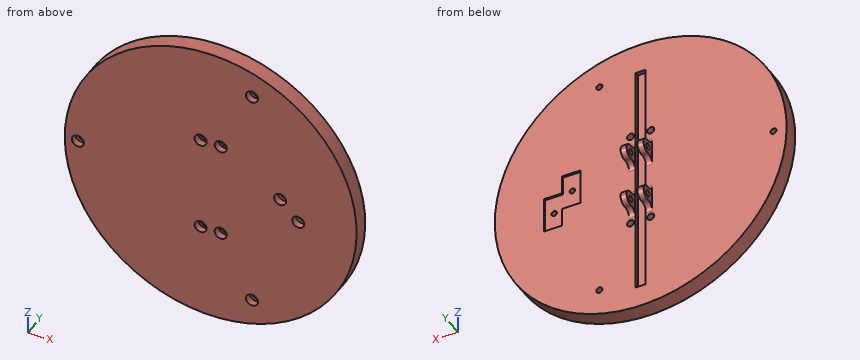
```python
from build123d import *

# Parameters (mm, degrees)
SKETCH_1_R             = 72.5
EXTRUDE_1_DEPTH        = 8
SKETCH_4_R             = 1.75
CUT_EXTRUDE_4_DEPTH    = 10
CUT_EXTRUDE_2_REACH    = 104.842
SKETCH_6_R             = 1.5
SKETCH_10_R            = 1.5
CUT_EXTRUDE_6_DEPTH    = 10
SKETCH_8_W             = 3
SKETCH_8_H             = 7
EXTRUDE_2_DEPTH        = 8
FILLET_1_R             = 3.5
SKETCH_9_R             = 1.5
CUT_EXTRUDE_5_DEPTH    = 106.675399219
FILLET_1_OF_MIRROR_1_R = 3.5
MIRROR_START           = -5.7
MIRROR_2_OUTLINE_R     = 1.5
MIRROR_2_DEPTH         = 3
SKETCH_11_R            = 1.35
CUT_EXTRUDE_7_DEPTH    = 103.842111997
SKETCH_12_W            = 9
SKETCH_12_H            = 18
CUT_EXTRUDE_8_DEPTH    = 1
SKETCH_7_R             = 3
CUT_EXTRUDE_3_DEPTH    = 3.5
SKETCH_14_W            = 5
SKETCH_14_H            = 1
SKETCH_14_H_2          = 117.17646446
CUT_EXTRUDE_9_DEPTH    = 2


# Read off the part's stored shape, not the designer's step: 镜向2
with BuildPart() as part:
    # 草图1 → 凸台-拉伸1 (new body)
    with BuildSketch(Plane(origin=(0, 0, 0), x_dir=(1, 0, 0), z_dir=(0, 1, 0))):
        with Locations(Location((0, 0, 0), (0, 0, 270))):
            Circle(SKETCH_1_R)
    extrude(amount=EXTRUDE_1_DEPTH)

    # 草图4 → 切除-拉伸4 (cut)
    with BuildSketch(Plane(origin=(0, 8, 0), x_dir=(1, 0, 0), z_dir=(0, 1, 0))):
        with Locations(Location((-5, -23, 0), (0, 0, 270))):
            Circle(SKETCH_4_R)
        with Locations(Location((-5, 25, 0), (0, 0, 270))):
            Circle(SKETCH_4_R)
        with Locations(Location((5, 25, 0), (0, 0, 270))):
            Circle(SKETCH_4_R)
        with Locations(Location((5, -23, 0), (0, 0, 270))):
            Circle(SKETCH_4_R)
    extrude(amount=-CUT_EXTRUDE_4_DEPTH, mode=Mode.SUBTRACT)

    # 草图6 → 切除-拉伸2 (cut, up to next)
    with BuildSketch(Plane(origin=(0, 8, 0), x_dir=(1, 0, 0), z_dir=(0, 1, 0)), mode=Mode.PRIVATE) as cut_extrude_2_sk1:
        with Locations(Location((20.5212086, -56.381557247, 0), (0, 0, 270))):
            Circle(SKETCH_6_R)
    cut_extrude_2_tool1 = extrude(cut_extrude_2_sk1.sketch, amount=-CUT_EXTRUDE_2_REACH, mode=Mode.PRIVATE) & part.part
    # 草图6 → 切除-拉伸2 (cut, up to next)
    with BuildSketch(Plane(origin=(0, 8, 0), x_dir=(1, 0, 0), z_dir=(0, 1, 0)), mode=Mode.PRIVATE) as cut_extrude_2_sk2:
        with Locations(Location((20.5212086, 56.381557247, 0), (0, 0, 270))):
            Circle(SKETCH_6_R)
    cut_extrude_2_tool2 = extrude(cut_extrude_2_sk2.sketch, amount=-CUT_EXTRUDE_2_REACH, mode=Mode.PRIVATE) & part.part
    add(cut_extrude_2_tool1.solids().sort_by_distance((20.521209, 8, 56.381557))[0], mode=Mode.SUBTRACT)
    add(cut_extrude_2_tool2.solids().sort_by_distance((20.521209, 8, -56.381557))[0], mode=Mode.SUBTRACT)

    # 草图10 → 切除-拉伸6 (cut)
    with BuildSketch(Plane(origin=(0, 8, 0), x_dir=(1, 0, 0), z_dir=(0, 1, 0))):
        with Locations(Location((-66, 0, 0), (0, 0, 270))):
            Circle(SKETCH_10_R)
    extrude(amount=-CUT_EXTRUDE_6_DEPTH, mode=Mode.SUBTRACT)

    # 草图8 → 凸台-拉伸2 (add)
    with BuildSketch(Plane(origin=(0, 8, 0), x_dir=(1, 0, 0), z_dir=(0, 1, 0))):
        with Locations((4.2, -10.911845751)):
            Rectangle(SKETCH_8_W, SKETCH_8_H)
    extrude_2 = extrude(amount=EXTRUDE_2_DEPTH)

    # 圆角1
    fillet_1_edges = [part.edges().sort_by_distance(p)[0] for p in [
        (4.2, 8, 7.411845751),
        (4.2, 8, 14.411845751),
    ]]
    fillet(fillet_1_edges, radius=FILLET_1_R)
    fillet_1_2_edges = [part.edges().sort_by_distance(p)[0] for p in [
        (4.2, 16, 7.411845751),
        (4.2, 16, 14.411845751),
    ]]
    fillet(fillet_1_2_edges, radius=FILLET_1_R - 0.0001)  # a hair under: the kernel refuses the full size

    # 草图9 → 切除-拉伸5 (cut, through all)
    with BuildSketch(Plane(origin=(2.7, 0, 0), x_dir=(0, 0, -1), z_dir=(1, 0, 0))):
        with Locations(Location((-10.975, 12, 0), (0, 0, 180))):
            Circle(SKETCH_9_R)
    cut_extrude_5 = extrude(amount=CUT_EXTRUDE_5_DEPTH, mode=Mode.SUBTRACT)

    # 镜向1: 凸台-拉伸2, 切除-拉伸5 across plane
    add(extrude_2.mirror(Plane.XY.offset(-2.025)))
    add(cut_extrude_5.mirror(Plane.XY.offset(-2.025)), mode=Mode.SUBTRACT)

    # 圆角1 of 镜向1
    fillet_1_of_mirror_1_edges = [part.edges().sort_by_distance(p)[0] for p in [
        (4.2, 8, -11.461845751),
        (4.2, 8, -18.461845751),
    ]]
    fillet(fillet_1_of_mirror_1_edges, radius=FILLET_1_OF_MIRROR_1_R)
    fillet_1_of_mirror_1_2_edges = [part.edges().sort_by_distance(p)[0] for p in [
        (4.2, 16, -11.461845751),
        (4.2, 16, -18.461845751),
    ]]
    fillet(fillet_1_of_mirror_1_2_edges, radius=FILLET_1_OF_MIRROR_1_R - 0.0001)  # a hair under: the kernel refuses the full size

    # 镜向2 outline → 镜向2 (add)
    # profile 1 of 2: a face of its own
    with BuildSketch(Plane.YZ.offset(MIRROR_START)):
        with BuildLine():
            ThreePointArc((11.5, -11.461845751), (9.025126266, -10.436719485), (8, -7.961845751))
            Line((8, -7.961845751), (8, -21.961845751))
            ThreePointArc((8, -21.961845751), (9.025126266, -19.486972017), (11.5, -18.461845751))
            Line((11.5, -18.461845751), (12.5, -18.461845751))
            ThreePointArc((12.5, -18.461845751), (14.974873734, -17.436719485), (16, -14.961845751))
            ThreePointArc((16, -14.961845751), (14.974873734, -12.486972017), (12.5, -11.461845751))
            Line((12.5, -11.461845751), (11.5, -11.461845751))
        make_face()
        with Locations((12, -15.025)):
            Circle(MIRROR_2_OUTLINE_R, mode=Mode.SUBTRACT)
    # profile 2 of 2: a face of its own
    with BuildSketch(Plane.YZ.offset(MIRROR_START)):
        with BuildLine():
            Line((12.5, 14.411845751), (11.5, 14.411845751))
            ThreePointArc((11.5, 14.411845751), (9.025126266, 15.436972017), (8, 17.911845751))
            Line((8, 17.911845751), (8, 3.911845751))
            ThreePointArc((8, 3.911845751), (9.025126266, 6.386719485), (11.5, 7.411845751))
            Line((11.5, 7.411845751), (12.5, 7.411845751))
            ThreePointArc((12.5, 7.411845751), (14.974873734, 8.436972017), (16, 10.911845751))
            ThreePointArc((16, 10.911845751), (14.974873734, 13.386719485), (12.5, 14.411845751))
        make_face()
        with Locations((12, 10.975)):
            Circle(MIRROR_2_OUTLINE_R, mode=Mode.SUBTRACT)
    extrude(amount=MIRROR_2_DEPTH)

    # 草图11 → 切除-拉伸7 (cut, through all)
    with BuildSketch(Plane(origin=(0, 8, 0), x_dir=(1, 0, 0), z_dir=(0, 1, 0))):
        with Locations(Location((34.508854567, -4.60948011, 0), (0, 0, 270))):
            Circle(SKETCH_11_R)
        with Locations(Location((43.508854567, 4.7, 0), (0, 0, 270))):
            Circle(SKETCH_11_R)
    extrude(amount=-CUT_EXTRUDE_7_DEPTH, mode=Mode.SUBTRACT)

    # 草图12 → 切除-拉伸8 (cut)
    with BuildSketch(Plane(origin=(0, 8, 0), x_dir=(1, 0, 0), z_dir=(0, 1, 0))):
        with Locations((43.508854567, 4.7)):
            Rectangle(SKETCH_12_W, SKETCH_12_H)
        with Locations((34.508854567, -4.60948011)):
            Rectangle(SKETCH_12_W, SKETCH_12_H)
    extrude(amount=-CUT_EXTRUDE_8_DEPTH, mode=Mode.SUBTRACT)

    # 草图7 → 切除-拉伸3 (cut)
    with BuildSketch(Plane.XZ):
        with Locations(Location((20.5212086, 56.381557247, 0), (0, 0, 270))):
            Circle(SKETCH_7_R)
        with Locations(Location((20.5212086, -56.381557247, 0), (0, 0, 270))):
            Circle(SKETCH_7_R)
        with Locations(Location((-5, 23, 0), (0, 0, 270))):
            Circle(SKETCH_7_R)
        with Locations(Location((5, 23, 0), (0, 0, 270))):
            Circle(SKETCH_7_R)
        with Locations(Location((5, -25, 0), (0, 0, 270))):
            Circle(SKETCH_7_R)
        with Locations(Location((-5, -25, 0), (0, 0, 270))):
            Circle(SKETCH_7_R)
        with Locations(Location((-66, 0, 0), (0, 0, 270))):
            Circle(SKETCH_7_R)
        with Locations(Location((43.508854567, -4.7, 0), (0, 0, 270))):
            Circle(SKETCH_7_R)
        with Locations(Location((34.508854567, 4.60948011, 0), (0, 0, 270))):
            Circle(SKETCH_7_R)
    extrude(amount=-CUT_EXTRUDE_3_DEPTH, mode=Mode.SUBTRACT)

    # 草图14 → 切除-拉伸9 (cut)
    with BuildSketch(Plane(origin=(0, 8, 0), x_dir=(1, 0, 0), z_dir=(0, 1, 0))):
        with Locations((0, 61.11323223)):
            Rectangle(SKETCH_14_W, SKETCH_14_H)
        with Locations((0, 2.025)):
            Rectangle(SKETCH_14_W, SKETCH_14_H_2)
        with Locations((0, -57.06323223)):
            Rectangle(SKETCH_14_W, SKETCH_14_H)
    extrude(amount=-CUT_EXTRUDE_9_DEPTH, mode=Mode.SUBTRACT)


solid = part.part
```
Design review of the part built by this model. Coordinates are the model's own, in mm. Give positions to 0.01 mm unless a question says otherwise; leave off trailing zeros. Order: outer loops, then holes, each group sorted by start corner. A loop starts at its lowest first (then second) coordinate and runs counter-clockwise, first axis right, second up. Notation, with made-up numbers: (59.25, 82.25) -> (86.25, 82.25) arc R19 ccw to (86.25, 118.25) -> close; hole circle Ø5 at (-19, -0.5). An arc over 180 degrees is marked (long way). Write each question's results on one line, items separated by ' | '. Start each with the question number.
Q1. Add section D-D on z = 23. Give the boundary of the cut face in (x, y) (3 decimals).
Q2. Add section B-B on x = 0. Give the boundary of the cut face in (y, z).
Q3. Add section C-C on z = 48. Give the boundary of the cut face in (x, y).
Q4. Wall thickness on L1, parallel to Z at x = 5.15, y = 12 (3 decimals); L2, parallel to X at y = 5.25, z = -25; L3, parallel to X at y = 12.25, z = 12.5: over which ranges is each line inside the solid? List them lowest first. Write a range as from..to.
Q5. For pin 1 (4 mm diameter, centred on y = 2, z = -23, fed in from -X); pin 2 (4 mm diameter, centred on y = 5, z = 9.5, fed in from -X); pin 3 (3 mm diameter, centred on x = 26.5, y = 4.5, fed in from +Z), all flat-tipped, find the tip position at first contact; note any pin that passes through.
Q6. Add section A-A on z = -25. Give the boundary of the cut face in (x, y), and give its area (3 significant figures).
Found:
1) outline: (-68.755, 0) -> (-8, 0) -> (-8, 3.5) -> (-6.75, 3.5) -> (-6.75, 8) -> (-68.755, 8) -> close; (-3.25, 3.5) -> (-2, 3.5) -> (-2, 0) -> (2, 0) -> (2, 3.5) -> (3.25, 3.5) -> (3.25, 8) -> (2.5, 8) -> (2.5, 6) -> (-2.5, 6) -> (-2.5, 8) -> (-3.25, 8) -> close; (6.75, 3.5) -> (8, 3.5) -> (8, 0) -> (68.755, 0) -> (68.755, 8) -> (6.75, 8) -> close
2) outline: (0, -72.5) -> (8, -72.5) -> (8, -61.61) -> (6, -61.61) -> (6, 57.56) -> (8, 57.56) -> (8, 72.5) -> (0, 72.5) -> close
3) outline: (-54.33, 0) -> (54.33, 0) -> (54.33, 8) -> (2.5, 8) -> (2.5, 6) -> (-2.5, 6) -> (-2.5, 8) -> (-54.33, 8) -> close
4) L1: z = -18.462..-16.525, -13.525..-11.462, 7.412..9.475, 12.475..14.412 | L2: x = -68.05..-6.75, -3.25..3.25, 6.75..68.05 | L3: x = -5.7..-2.7, 2.7..5.7
5) pin 1: stops at x = -69.39 | pin 2: stops at x = -72.11 | pin 3: stops at z = 68.05
6) outline: (-68.05, 0) -> (-8, 0) -> (-8, 3.5) -> (-6.75, 3.5) -> (-6.75, 8) -> (-68.05, 8) -> close; (-3.25, 3.5) -> (-2, 3.5) -> (-2, 0) -> (2, 0) -> (2, 3.5) -> (3.25, 3.5) -> (3.25, 8) -> (2.5, 8) -> (2.5, 6) -> (-2.5, 6) -> (-2.5, 8) -> (-3.25, 8) -> close; (6.75, 3.5) -> (8, 3.5) -> (8, 0) -> (68.05, 0) -> (68.05, 8) -> (6.75, 8) -> close | area: 1,010 mm2
